```python
from build123d import *

# Parameters (mm, degrees)
SKETCH1_W            = 160.5788
SKETCH1_H            = 37.338
BOSS_EXTRUDE1_DEPTH  = 12.7
SKETCH2_W            = 157.5308
SKETCH2_H            = 34.29
CUT_EXTRUDE3_DEPTH   = 11.049
FILLET1_R            = 2.54
FILLET2_R            = 1.27
CUT_EXTRUDE4_REACH   = 164.158
SKETCH4_W            = 159.0548
SKETCH4_H            = 35.814
CUT_EXTRUDE5_DEPTH   = 1.778
FILLET3_R            = 1.524
SKETCH5_W            = 5.08
SKETCH5_H            = 0.762
BOSS_EXTRUDE2_DEPTH  = 7.62
SKETCH6_W            = 0.762
SKETCH6_H            = 2.032
BOSS_EXTRUDE3_DEPTH  = 13.589
LPATTERN1_COUNT      = 2
LPATTERN1_PITCH      = 101.6
LPATTERN1_COUNT_DIR2 = 2
LPATTERN1_PITCH_DIR2 = 32.258
CUT_EXTRUDE6_REACH   = 133.936
SKETCH8_W            = 3.81
SKETCH8_H            = 2.032
BOSS_EXTRUDE4_DEPTH  = 14.859
BOSS_EXTRUDE9_DEPTH  = 3.81
FILLET4_R            = 0.254
FILLET4_OF_MIRROR2_R = 0.254
SKETCH10_R           = 14.732
SKETCH10_R_2         = 1.905
CUT_EXTRUDE7_DEPTH   = 85.490976307


with BuildPart() as part:
    # Sketch1 → Boss-Extrude1 (new body)
    with BuildSketch(Plane(origin=(0, 0, 0), x_dir=(1, 0, 0), z_dir=(0, 1, 0))):
        Rectangle(SKETCH1_W, SKETCH1_H)
    extrude(amount=BOSS_EXTRUDE1_DEPTH)

    # Sketch2 → Cut-Extrude3 (cut)
    with BuildSketch(Plane(origin=(0, 12.7, 0), x_dir=(1, 0, 0), z_dir=(0, 1, 0))):
        Rectangle(SKETCH2_W, SKETCH2_H)
    extrude(amount=-CUT_EXTRUDE3_DEPTH, mode=Mode.SUBTRACT)

    # Fillet1
    fillet1_edges = [part.edges().sort_by_distance(p)[0] for p in [
        (0, 0, 18.669),
        (-80.2894, 0, 0),
        (0, 0, -18.669),
        (80.2894, 0, 0),
        (80.2894, 6.35, 18.669),
        (-80.2894, 6.35, 18.669),
        (-80.2894, 6.35, -18.669),
        (80.2894, 6.35, -18.669),
    ]]
    fillet(fillet1_edges, radius=FILLET1_R)

    # Fillet2
    fillet2_edges = [part.edges().sort_by_distance(p)[0] for p in [
        (-78.7654, 7.1755, -17.145),
        (-78.7654, 7.1755, 17.145),
        (78.7654, 7.1755, 17.145),
        (78.7654, 7.1755, -17.145),
    ]]
    fillet(fillet2_edges, radius=FILLET2_R)

    # Sketch3 → Cut-Extrude4 (cut, up to next)
    with BuildSketch(Plane.ZY.offset(80.2894), mode=Mode.PRIVATE) as cut_extrude4_sk1:
        with BuildLine():
            Line((3.81, 3.8633146), (-3.81, 3.8633146))
            ThreePointArc((-3.81, 3.8633146), (-7.366, 7.4193146), (-3.81, 10.9753146))
            Line((-3.81, 10.9753146), (3.81, 10.9753146))
            ThreePointArc((3.81, 10.9753146), (7.366, 7.4193146), (3.81, 3.8633146))
        make_face()
    cut_extrude4_tool1 = extrude(cut_extrude4_sk1.sketch, amount=-CUT_EXTRUDE4_REACH, mode=Mode.PRIVATE) & part.part
    add(cut_extrude4_tool1.solids().sort_by_distance((-80.2894, 7.419315, 0))[0], mode=Mode.SUBTRACT)

    # Sketch4 → Cut-Extrude5 (cut)
    with BuildSketch(Plane(origin=(0, 12.7, 0), x_dir=(1, 0, 0), z_dir=(0, 1, 0))):
        Rectangle(SKETCH4_W, SKETCH4_H)
    extrude(amount=-CUT_EXTRUDE5_DEPTH, mode=Mode.SUBTRACT)

    # Fillet3
    fillet3_edges = [part.edges().sort_by_distance(p)[0] for p in [
        (-79.5274, 11.811, 17.907),
        (-79.5274, 11.811, -17.907),
        (79.5274, 11.811, -17.907),
        (79.5274, 11.811, 17.907),
    ]]
    fillet(fillet3_edges, radius=FILLET3_R)

    # Sketch5 → Boss-Extrude2 (add)
    with BuildSketch(Plane(origin=(0, 10.922, 0), x_dir=(1, 0, 0), z_dir=(0, 1, 0))):
        with Locations((-74.9554, -17.526)):
            Rectangle(SKETCH5_W, SKETCH5_H)
    extrude(amount=BOSS_EXTRUDE2_DEPTH)

    # Sketch6 → Boss-Extrude3 (add)
    with BuildSketch(Plane(origin=(0, 1.651, 0), x_dir=(1, 0, 0), z_dir=(0, 1, 0))):
        with Locations((-52.9844, 16.129)):
            Rectangle(SKETCH6_W, SKETCH6_H)
    boss_extrude3 = extrude(amount=BOSS_EXTRUDE3_DEPTH)

    # LPattern1: Boss-Extrude3 2 × 2
    with Locations(*[(i * LPATTERN1_PITCH, 0, j * LPATTERN1_PITCH_DIR2) for i in range(LPATTERN1_COUNT) for j in range(LPATTERN1_COUNT_DIR2) if (i, j) != (0, 0)]):
        add(boss_extrude3)

    # Cut-Extrude6: up to this face of the body (flat: up to its plane)
    cut_extrude6_end = Plane(part.part.faces().sort_by_distance((-53.3654, 8.4455, -16.129))[0])
    # Sketch7 → Cut-Extrude6 (cut, up to the picked face)
    with BuildSketch(Plane(origin=(48.9966, 0, 0), x_dir=(0, 0, -1), z_dir=(1, 0, 0)), mode=Mode.PRIVATE) as cut_extrude6_sk1:
        Polygon((17.145, 10.922), (15.494, 15.24), (17.145, 15.24), align=None)
    cut_extrude6_tool1 = split(extrude(cut_extrude6_sk1.sketch, amount=-CUT_EXTRUDE6_REACH, mode=Mode.PRIVATE), bisect_by=cut_extrude6_end, keep=Keep.BOTH, mode=Mode.PRIVATE)
    cut_extrude6 = cut_extrude6_tool1.solids().sort_by(Axis((48.9966, 13.800667, -16.594667), (-1, 0, 0)))[0]
    add(cut_extrude6, mode=Mode.SUBTRACT)

    # Mirror1: Cut-Extrude6 across plane
    add(cut_extrude6.mirror(Plane.XY), mode=Mode.SUBTRACT)

    # Sketch8 → Boss-Extrude4 (add)
    with BuildSketch(Plane(origin=(0, 1.651, 0), x_dir=(1, 0, 0), z_dir=(0, 1, 0))):
        with Locations((0, -16.129)):
            Rectangle(SKETCH8_W, SKETCH8_H)
        with Locations((0, 16.129)):
            Rectangle(SKETCH8_W, SKETCH8_H)
    extrude(amount=BOSS_EXTRUDE4_DEPTH)

    # Sketch9 → Boss-Extrude9 (add)
    with BuildSketch(Plane(origin=(1.905, 0, 0), x_dir=(0, 0, -1), z_dir=(1, 0, 0))):
        Polygon((-15.113, 16.51), (-17.907, 16.51), (-15.113, 18.542), align=None)
    boss_extrude9 = extrude(amount=-BOSS_EXTRUDE9_DEPTH)

    # Fillet4
    fillet4_edges = [part.edges().sort_by_distance(p)[0] for p in [
        (0, 18.542, 15.113),
    ]]
    fillet(fillet4_edges, radius=FILLET4_R)

    # Mirror2: Boss-Extrude9 across plane
    add(boss_extrude9.mirror(Plane.XY))

    # Fillet4 of Mirror2
    fillet4_of_mirror2_edges = [part.edges().sort_by_distance(p)[0] for p in [
        (0, 18.542, -15.113),
    ]]
    fillet(fillet4_of_mirror2_edges, radius=FILLET4_OF_MIRROR2_R)

    # Sketch10 → Cut-Extrude7 (cut, through all)
    with BuildSketch(Plane.XZ):
        with Locations(Location((0, 0, 0), (0, 0, 270))):
            Circle(SKETCH10_R)
        with Locations(Location((-20.193, 0, 0), (0, 0, 270))):
            Circle(SKETCH10_R_2)
        with Locations(Location((20.193, 0, 0), (0, 0, 270))):
            Circle(SKETCH10_R_2)
    extrude(amount=-CUT_EXTRUDE7_DEPTH, mode=Mode.SUBTRACT)


solid = part.part
```
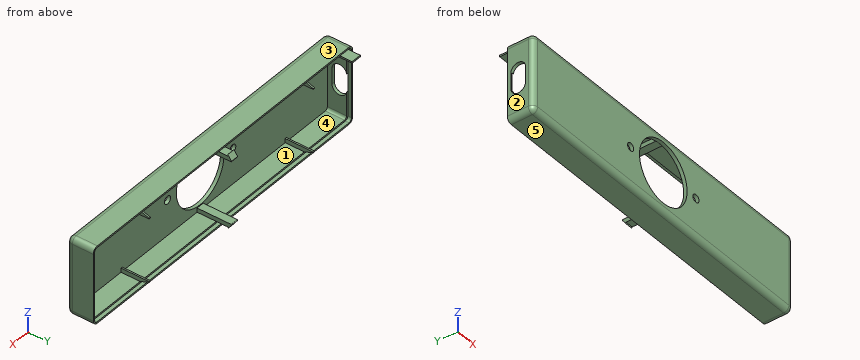
Work out the finished part from the listing and answer in its coordinate system (mm). Face numbers are marked on the shaded views. A direction names the side the tool comes from. Round coordinates to 2 decimals unless told otherwise and drop trailing zeros. Write each loop counter-clockwise with the first axis right and the second up, starting at its lowest first coordinate (ties: lowest second). Pieces come first, ordered by that corner, then holes. Notation, with made-up numbers: (33.25, -31.5) - (68.25, -31.5) arc R26 ccw to (68.25, 0.5) - close; hole circle Ø5 at (46, 47.5). An arc over 180 degrees is marked (long way). Return JSON: item names as keys, results as strings. Group by question number.
Q1. The mould has two halves that part along Z. Classify the marked faces 1, 2 and 3: released by +Z, released by -Z, zero draft, split by the parting line, or undercut.
Q2. The part is cut by section A-A on x = 0. Write down the section's boundary in (y, z) (3 decimals).
Q3. For the marked faces 4 and 5, determine the directions among +Z, -Z, +X, -X, +Y, -Y from which every point of the face is accessible in a straight line to the end or side of a thin tool.
Q4. The part is cut by section D-D on x = -55.5. Write down the section's boundary in (y, z) (3 decimals), then the cut area to 3 significant figures.
Q5. Find the intervals of material crossed by L1, parallel to X at y = 6.75, z = 16 (3 decimals); L2, parallel to Z at x = -6, y = 11; L3, parallel to Z at x = 27.5, y = 6 (3 decimals), in increasing order.
Q6. The part is cut by section B-B on z = 0. Write down the section's boundary in (x, y).
Q7. Each of these flat-tipped pins is pushed along its axis until it touches: pin 1 Ø1.5 at (x, z) = (-48, 6) entering from +Y; pin 2 Ø0.6 at (x, z) = (0.5, -17.5) entering from -Y; pin 3 Ø1.4 at (y, z) = (9.5, -17) entering from -X. Where does it stop, or does it pass through?
Q8. The part is cut by section C-C on z = 13. Write down the section's boundary in (x, y), then the cut area to 3 significant figures.
Solved:
{
 "1": {"face 1": "undercut", "face 2": "zero draft", "face 3": "released by +Z"},
 "2": {"outline": "(0, -16.129) arc R2.54 ccw to (2.54, -18.669) - (12.7, -18.669) - (12.7, -17.907) - (10.922, -17.907) - (10.922, -17.145) - (16.51, -17.145) - (16.51, -17.907) - (18.249, -15.516) arc R0.254 ccw to (18.043, -15.113) - (1.651, -15.113) - (1.651, -14.732) - (0, -14.732) - close; (0, 14.732) - (1.651, 14.732) - (1.651, 15.113) - (18.043, 15.113) arc R0.254 ccw to (18.249, 15.516) - (16.51, 17.907) - (16.51, 17.145) - (10.922, 17.145) - (10.922, 17.907) - (12.7, 17.907) - (12.7, 18.669) - (2.54, 18.669) arc R2.54 ccw to (0, 16.129) - close"},
 "3": {"face 4": "+Y", "face 5": "-Z, +X, -X, +Y, -Y"},
 "4": {"outline": "(0, -16.129) arc R2.54 ccw to (2.54, -18.669) - (12.7, -18.669) - (12.7, -17.907) - (10.922, -17.907) - (10.922, -17.145) - (1.651, -17.145) - (1.651, 17.145) - (10.922, 17.145) - (10.922, 17.907) - (12.7, 17.907) - (12.7, 18.669) - (2.54, 18.669) arc R2.54 ccw to (0, 16.129) - close", "area": "89.8 mm²"},
 "5": {"L1": "-80.289 to -78.759, -53.365 to -52.603, -1.905 to 1.905, 48.235 to 48.997, 78.759 to 80.289", "L2": "-18.67 to -17.91, 17.91 to 18.67", "L3": "-18.669 to -17.145, 17.145 to 18.669"},
 "6": {"outline": "(-80.29, 2.54) arc R2.54 ccw to (-77.75, 0) - (-22.1, 0) - (-22.1, 1.65) - (-78.77, 1.65) - (-78.77, 3.86) - (-80.29, 3.86) - close; (-80.29, 10.98) - (-79.53, 10.98) - (-79.53, 12.7) - (-80.29, 12.7) - close; (-18.29, 0) - (-14.73, 0) - (-14.73, 1.65) - (-18.29, 1.65) - close; (14.73, 0) - (18.29, 0) - (18.29, 1.65) - (14.73, 1.65) - close; (22.1, 0) - (77.75, 0) arc R2.54 ccw to (80.29, 2.54) - (80.29, 12.7) - (79.53, 12.7) - (79.53, 10.92) - (78.77, 10.92) - (78.77, 1.65) - (22.1, 1.65) - close"},
 "7": {"pin 1": "y = 1.65", "pin 2": "y = 0.24", "pin 3": "x = -80.28"},
 "8": {"outline": "(-80.29, 2.54) arc R2.54 ccw to (-77.75, 0) - (-6.93, 0) - (-6.93, 1.65) - (-78.77, 1.65) - (-78.77, 10.92) - (-79.53, 10.92) - (-79.53, 12.7) - (-80.29, 12.7) - close; (6.93, 0) - (77.75, 0) arc R2.54 ccw to (80.29, 2.54) - (80.29, 12.7) - (79.53, 12.7) - (79.53, 10.92) - (78.77, 10.92) - (78.77, 1.65) - (6.93, 1.65) - close", "area": "270 mm²"}
}
